Can you work these out from the model? Positions are in its coordinate system, mm. A direction names the side the tool comes from. Give positions to 0.01 mm unless a question says otherwise; leave off trailing zeros. Loops run counter-clockwise (first coordinate to the right, second up) from the corner with the lowest first, then second, coordinate; pieces in that order, holes last. Notation, with made-up numbers: (5, 23.25) - (41, 23.25) arc R29 ccw to (41, 47.25) - close; hole circle Ø8 at (19.25, 6.5). An arc over 180 degrees is marked (long way). Answer as a JSON object with one key per item and string values. Group by question number.
Item 1: Which directions (+Z, -Z, +X, -X, +Y, -Y) give clear straight access to the entire face, cutting with the end or side of a thin tool? Please do faces 1 (the cylindrical face through (53.647, 3.729, 3.217)), 2 (the flat face through (40.042, 6.229, -7.007)), 3 (the flat face through (-18, 2, 0)), 4 (the flat face through (-18, 7, -5.375)).
Item 2: Suppose I cut it at A-A on x = -28.5. Write out the boundary of the cut face in (y, z) (3 decimals), and give its area (3 significant figures).
Item 3: Suppose I cut it at C-C on y = 7. Write out the boundary of the cut face in (x, z) (3 decimals), and give its area (3 significant figures).
Item 4: Suppose I cut it at D-D on x = 3.5. Write out the boundary of the cut face in (y, z), and give its area (3 significant figures).
Item 5: Thinking about a two-plate mould opening in X: for faces 5 (the flat face through (-37.67, 7, 0)), 6 (the flat face through (-18, 7, 5.375)), 7 (the flat face through (27.12, 7.15, 0.06)), 8 (the flat face through (40.042, 6.229, 7.007)), which applies, pulls with the +X half, pulls with the -X half, needs draft (parallel to the pull), parting line crosses it, or undercut?
Item 6: Will these pins go through, and if not, where does the flat tip stop? pin 1 (4 mm diameter, centred on x = -9, y = 6.5, fed in from +Z) (3 decimals); pin 2 (1.5 mm diameter, centred on x = -24.5, y = 12, fed in from -Z) (3 decimals); pin 3 (4.5 mm diameter, centred on x = -10.5, z = 0.5, fed in from +Y).
Item 7: Please list where these lines run through material, in increasing order: L1, parallel to Z at x = 4, y = 11.25; L2, parallel to Y at x = -10, z = -1; L3, parallel to Y at x = 27, z = -3.75.
from build123d import *
from OCP.BRepFilletAPI import BRepFilletAPI_MakeChamfer

# Parameters (mm, degrees)
BOSS_EXTRUDE1_DEPTH = 7.5
SKETCH3_W           = 10.75
SKETCH3_H           = 9.75
BOSS_EXTRUDE2_DEPTH = 37.67
CUT_EXTRUDE9_START  = -3
CUT_EXTRUDE9_DEPTH  = 9
FILLET1_R           = 4.5
CHAMFER1_SIZE       = 1
CHAMFER1_SIZE2      = 0.867711944
CHAMFER3_SIZE       = 0.75


with BuildPart() as part:
    # Sketch2 → Boss-Extrude1 (new, symmetric)
    with BuildSketch(Plane.XY):
        Polygon((0, 0), (80, 0), (0, 13.5), align=None)
    extrude(amount=BOSS_EXTRUDE1_DEPTH, both=True)

    # Sketch3 → Boss-Extrude2 (add)
    with BuildSketch(Plane.ZY):
        with Locations((0, 6.875)):
            Rectangle(SKETCH3_W, SKETCH3_H)
    extrude(amount=BOSS_EXTRUDE2_DEPTH)

    # Sketch4 → Cut-Extrude9 (cut)
    with BuildSketch(Plane.XY.offset(7.5).offset(CUT_EXTRUDE9_START)):
        Polygon((55, 4.21875), (0, 13.5), (0, 11.725257914), (55, 2.444007914), align=None)
    extrude(amount=-CUT_EXTRUDE9_DEPTH, mode=Mode.SUBTRACT)

    # Fillet1
    fillet1_edges = [part.edges().sort_by_distance(p)[0] for p in [
        (55, 3.331378957, 4.5),
        (55, 3.331378957, -4.5),
    ]]
    fillet(fillet1_edges, radius=FILLET1_R - 0.0001)  # a hair under: the kernel refuses the full size

    # Chamfer1: one chamfer whose edges measure the first distance from different faces: ONE call of the kernel's chamfer builder (chamfer() names one face for all edges)
    chamfer1_edges_1 = [part.edges().sort_by_distance(p)[0] for p in [
        (40, 6.75, 7.5),
        (40, 6.75, -7.5),
    ]]
    chamfer1_edges_2 = [part.edges().sort_by_distance(p)[0] for p in [
        (80, 0, 0),
    ]]
    chamfer1_side_2 = [part.faces().sort_by_distance(p)[0] for p in [
        (40, 0, 0),
    ]]
    chamfer1 = BRepFilletAPI_MakeChamfer(part.part.solid().wrapped)
    for e in chamfer1_edges_1:
        chamfer1.Add(CHAMFER1_SIZE, e.wrapped)
    for e in chamfer1_edges_2:
        chamfer1.Add(CHAMFER1_SIZE, CHAMFER1_SIZE2, e.wrapped, chamfer1_side_2[0].wrapped)  # the first distance lies on this face
    add(Compound.cast(chamfer1.Shape()), mode=Mode.REPLACE)

    # Chamfer3
    chamfer3_edges = [part.edges().sort_by_distance(p)[0] for p in [
        (-18.835, 11.75, -5.375),
        (-18.835, 2, -5.375),
        (-18.835, 2, 5.375),
        (-18.835, 11.75, 5.375),
        (-37.67, 6.875, -5.375),
        (-37.67, 2, 0),
        (-37.67, 6.875, 5.375),
        (-37.67, 11.75, 0),
    ]]
    chamfer(chamfer3_edges, length=CHAMFER3_SIZE)


solid = part.part
Worked out:
{
 "1": {"face 1": "+Y", "face 2": "-Z, +X, +Y", "face 3": "+Z, -Z, -X, -Y", "face 4": "-Z, -X, +Y, -Y"},
 "2": {"outline": "(2, -4.625) - (2.75, -5.375) - (11, -5.375) - (11.75, -4.625) - (11.75, 4.625) - (11, 5.375) - (2.75, 5.375) - (2, 4.625) - close", "area": "104 mm2"},
 "3": {"outline": "(-37.67, -4.625) - (-36.92, -5.375) - (0, -5.375) - (0, -7.5) - (32.509, -7.5) - (38.519, -6.5) - (38.519, -4.5) - (28.002, -4.5) - (28.002, 4.5) - (38.519, 4.5) - (38.519, 6.5) - (32.509, 7.5) - (0, 7.5) - (0, 5.375) - (-36.92, 5.375) - (-37.67, 4.625) - close", "area": "882 mm2"},
 "4": {"outline": "(0, -7.5) - (11.9, -7.5) - (12.91, -6.5) - (12.91, -4.5) - (11.13, -4.5) - (11.13, 4.5) - (12.91, 4.5) - (12.91, 6.5) - (11.9, 7.5) - (0, 7.5) - close", "area": "177 mm2"},
 "5": {"face 5": "pulls with the -X half", "face 6": "needs draft", "face 7": "undercut", "face 8": "pulls with the +X half"},
 "6": {"pin 1": "stops at z = 5.375", "pin 2": "stops at z = -5.125", "pin 3": "stops at y = 11.75"},
 "7": {"L1": "z = -7.5 to -4.5, 4.5 to 7.5", "L2": "y = 2 to 11.75", "L3": "y = 0 to 7.17"}
}
